from build123d import *

# Parameters (mm, degrees)
SALIENTE_EXTRUIR1_DEPTH = 7.5
SALIENTE_EXTRUIR2_DEPTH = 15
CROQUIS7_R              = 3.5
CORTAR_EXTRUIR4_DEPTH   = 10.5
CORTAR_EXTRUIR5_START   = -3
CORTAR_EXTRUIR5_DEPTH   = 10
CHAFL_N4_SIZE           = 4
CHAFL_N5_SIZE           = 0.8


with BuildPart() as part:
    # Croquis1 → Saliente-Extruir1 (new body, symmetric)
    with BuildSketch(Plane.XY):
        with BuildLine():
            Line((-8.9, 4), (-4.936786437, 7.963213563))
            ThreePointArc((-4.936786437, 7.963213563), (-4.038051049, 5.609646436), (-2.1, 4))
            Line((-2.1, 4), (0, 4))
            Line((0, 4), (0, -4))
            ThreePointArc((0, -4), (-4.823611651, -3.031815583), (-8.9, -0.277243303))
            Line((-8.9, -0.277243303), (-8.9, 4))
        make_face()
    extrude(amount=SALIENTE_EXTRUIR1_DEPTH, both=True)

    # Croquis6 → Saliente-Extruir2 (add, through all)
    with BuildSketch(Plane(origin=(0, 0, -7.5), x_dir=(-1, 0, 0), z_dir=(0, 0, -1))):
        Polygon((0, 4), (-1.5, 5.5), (-22.5, 5.5), (-22.5, -4), (0, -4), align=None)
    extrude(amount=-SALIENTE_EXTRUIR2_DEPTH)

    # Croquis7 → Cortar-Extruir4 (cut, through all)
    with BuildSketch(Plane(origin=(0, 5.5, 0), x_dir=(1, 0, 0), z_dir=(0, 1, 0))):
        with Locations((15, 0)):
            Circle(CROQUIS7_R)
    extrude(amount=-CORTAR_EXTRUIR4_DEPTH, mode=Mode.SUBTRACT)

    # Croquis8 → Cortar-Extruir5 (cut)
    with BuildSketch(Plane(origin=(0, 5.5, 0), x_dir=(1, 0, 0), z_dir=(0, 1, 0)).offset(CORTAR_EXTRUIR5_START)):
        Polygon((15, 5.658032638), (10.1, 2.829016319), (10.1, -2.829016319), (15, -5.658032638), (19.9, -2.829016319), (19.9, 2.829016319), align=None)
    extrude(amount=-CORTAR_EXTRUIR5_DEPTH, mode=Mode.SUBTRACT)

    # Chaflán4
    chafl_n4_edges = [part.edges().sort_by_distance(p)[0] for p in [
        (22.5, 0.75, 7.5),
        (22.5, 0.75, -7.5),
    ]]
    chamfer(chafl_n4_edges, length=CHAFL_N4_SIZE)

    # Chaflán5
    chafl_n5_edges = [part.edges().sort_by_distance(p)[0] for p in [
        (11.5, 5.5, 0),
        (12.55, -4, -4.243524479),
        (10.1, -4, 0),
        (12.55, -4, 4.243524479),
        (17.45, -4, 4.243524479),
        (19.9, -4, 0),
        (17.45, -4, -4.243524479),
    ]]
    chamfer(chafl_n5_edges, length=CHAFL_N5_SIZE)


solid = part.part
Part model, mm, in its own coordinate system. A direction names the side the tool comes from. Coordinates: 2 decimals unless noted, no trailing zeros. Order: outer loops, then holes, each group sorted by start corner. A loop starts at its lowest first (then second) coordinate and runs counter-clockwise, first axis right, second up. Notation, with made-up numbers: M 32.5,85 L 82.5,85 A20 cw 82.5,108 Z; hole C -39,13.25 d6. An arc over 180 degrees is marked long. One line per question, with ' | ' between items.
Q1. Slice it at B-B (z = 0). Give the cut face in (x, y).
A:
outline: M -8.9,-0.28 A12.5 ccw 0,-4 L 9.3,-4 L 10.1,-3.2 L 10.1,2.5 L 11.5,2.5 L 11.5,4.7 L 10.7,5.5 L 1.5,5.5 L 0,4 L -2.1,4 A4.97 cw -4.94,7.96 L -8.9,4 Z; M 18.5,2.5 L 19.9,2.5 L 19.9,-3.2 L 20.7,-4 L 22.5,-4 L 22.5,5.5 L 19.3,5.5 L 18.5,4.7 Z
Q2. Two-plate mould, pull along Z, no slides. Class faces 4 (the face through (9.7, -3.6, 0)), 5 (the face through (21, 1, 5)), 6 (the face through (9, -4, 0)): +Z half, -Z half, draft (parallel to the pull), parting line (faces both ways), or undercut.
A:
face 4: undercut | face 5: +Z half | face 6: draft
Q3. Pin check, flat tips, straight feed: P1, Ø1.5, axis at x = 15, z = 4, coming from the -Y side; P2, Ø2.5, axis at x = -1, z = 0.5, coming from the +Y side; P3, Ø9, axis at x = 15, z = 0, coming from the +Y side. Stop position of each tip, or through.
A:
P1: stops at y = 2.5 | P2: stops at y = 4.25 | P3: stops at y = 5.5
Q4. Slice it at D-D (y = -2.75). Give the cut face in (x, z).
A:
outline: M -5.45,-7.5 L 18.5,-7.5 L 22.5,-3.5 L 22.5,3.5 L 18.5,7.5 L -5.45,7.5 Z; hole M 10.1,-2.83 L 15,-5.66 L 19.9,-2.83 L 19.9,2.83 L 15,5.66 L 10.1,2.83 Z
Q5. Slice it at A-A (y = 2). Give the cut face in (x, z), and give its area (3 significant figures).
A:
outline: M -8.9,-7.5 L 18.5,-7.5 L 22.5,-3.5 L 22.5,3.5 L 18.5,7.5 L -8.9,7.5 Z; hole M 10.1,-2.83 L 15,-5.66 L 19.9,-2.83 L 19.9,2.83 L 15,5.66 L 10.1,2.83 Z | area: 372 mm^2
Q6. Drill centre lines: line 1 (Z direction, x = 15, y = 4.1); line 2 (X direction, y = 3.3, z = 0); line 3 (X direction, y = 4.75, z = 3). Where is each one in solid material? Low to high.
A:
line 1: z = -7.5 to -3.5, 3.5 to 7.5 | line 2: x = -8.9 to 11.5, 18.5 to 22.5 | line 3: x = -8.15 to -3.26, 0.75 to 13.1, 16.9 to 22.5
Q7. 3-axis set-ups, long thin cutter, end or side, ignore diameter. For faces 1 (the face through (1, 5, 0)), 2 (the face through (12.313, -3.594, -4.562)), 3 (the face through (-8.9, 2, 0)): which of +Z, -Z, +X, -X, +Y, -Y reach the whole face in a straight line?
A:
face 1: +Z, -Z, +Y | face 2: -Y | face 3: +Z, -Z, -X, +Y, -Y
Q8. Slice it at C-C (z = 4.75). Give the cut face in (x, y), and give its area (3 significant figures).
A:
outline: M -8.9,-0.28 A12.5 ccw 0,-4 L 11.83,-4 L 13.43,-3.2 L 13.43,2.5 L 16.57,2.5 L 16.57,-3.2 L 18.17,-4 L 21.25,-4 L 21.25,5.5 L 1.5,5.5 L 0,4 L -2.1,4 A4.97 cw -4.94,7.96 L -8.9,4 Z | area: 251 mm^2
